Check sheet for the modelled part. Datum: model origin and axes. Units: mm. A direction names the side the tool comes from. Give positions to 0.01 mm unless a question says otherwise; leave off trailing zeros. Write each loop counter-clockwise with the first axis right and the second up, starting at its lowest first coordinate (ties: lowest second). Pieces come first, ordered by that corner, then holes. Notation, with made-up numbers: (7.5, 52.25) -> (59.5, 52.25) arc R30 cw to (59.5, 77.25) -> close; hole circle Ø5 at (8.5, 31). An arc over 180 degrees is marked (long way). Use a Markdown table: item, result. Add a question column.
1. Cross-section at D-D (y = 160.5). Enter the section's corners in (x, z), then the cut area to 3 significant figures.
2. Cross-section at A-A (z = 0). Enter the section's corners in (x, y).
3. Gauge pin test, flat ends, axial feed: P1, Ø1.5, axis at x = 70, y = 53, coming from the +Z side; P2, Ø3, axis at x = -80, y = 63.5, coming from the -Z side; P3, Ø5.5, axis at x = -80, z = 46.5, coming from the +Y side; P4, Ø1.5, axis at x = 81.5, z = 18, coming from the -Y side. Record the tip position at first contact, or that the pin passes through.
4. Cross-section at B-B (x = 0). Enter the section's corners in (y, z).
5. Cross-section at C-C (y = 209). Enter the section's corners in (x, z), then the cut area to 3 significant figures.
6. Release check for a two-part mould opening along X. For faces 1 (the cylindrical face through (-15.456, 224.956, -20.157)), 2 (the cylindrical face through (0.372, 29.58, -118.492)), 3 (the flat face through (-72.335, 63.131, 41.852)), 4 (the cylindrical face through (77.38, 29.58, -43.77)) record: released by +X, released by -X, zero draft, split by the parting line, or undercut.
7. Set-up check for faces 5 (the flat face through (-67, 30, 71.947)), 6 (the flat face through (66, 30, 71.947)), 7 (the flat face through (-81, 66.35, 46)), 8 (the cylindrical face through (22.89, 153.67, -72.68)): record each of +Z, -Z, +X, -X, +Y, -Y from which the full face is reachable in a straight line by a thin tool's end or side.
8. Scan lines: probe 1 along X at (y, z) = (219.5, 0); probe 2 along Y at (x, z) = (-63, 53.5); probe 3 along Y at (x, z) = (-7, -4). Record each from-to range of solid material in increasing order. Write a range as [from, to].
from build123d import *

# Parameters (mm, degrees)
BOSS_EXTRUDE1_DEPTH = 60
BOSS_EXTRUDE2_DEPTH = 6.35
SKETCH3_R           = 76.2
BOSS_EXTRUDE3_DEPTH = 250
SKETCH4_R           = 25.4
CUT_EXTRUDE1_DEPTH  = 50.8


with BuildPart() as part:
    # Sketch1 → Boss-Extrude1 (new body)
    with BuildSketch(Plane(origin=(0, 0, 0), x_dir=(1, 0, 0), z_dir=(0, 1, 0))):
        with BuildLine():
            ThreePointArc((-36.198972693, 81.196332281), (-76.989658396, 44.45), (-88.417572796, -9.248936198))
            Line((-88.417572796, -9.248936198), (-102.619500233, -33.847396084))
            ThreePointArc((-102.619500233, -33.847396084), (-102.619500233, -59.247396084), (-80.622454977, -71.947396084))
            Line((-80.622454977, -71.947396084), (-52.218600103, -71.947396084))
            ThreePointArc((-52.218600103, -71.947396084), (0, -88.9), (52.218600103, -71.947396084))
            Line((52.218600103, -71.947396084), (80.622454977, -71.947396084))
            ThreePointArc((80.622454977, -71.947396084), (102.619500233, -59.247396084), (102.619500233, -33.847396084))
            Line((102.619500233, -33.847396084), (88.417572796, -9.248936198))
            ThreePointArc((88.417572796, -9.248936198), (76.989658396, 44.45), (36.198972693, 81.196332281))
            Line((36.198972693, 81.196332281), (21.997045256, 105.794792168))
            ThreePointArc((21.997045256, 105.794792168), (0, 118.494792168), (-21.997045256, 105.794792168))
            Line((-21.997045256, 105.794792168), (-36.198972693, 81.196332281))
        make_face()
        with BuildLine():
            ThreePointArc((-75.786490968, -7.927659598), (-65.991135768, 38.1), (-31.02769088, 69.596856241))
            ThreePointArc((-31.02769088, 69.596856241), (0, 76.2), (31.02769088, 69.596856241))
            ThreePointArc((31.02769088, 69.596856241), (63.916938463, 41.485720163), (76.2, 0))
            ThreePointArc((76.2, 0), (76.096552523, -3.969218324), (75.786490968, -7.927659598))
            ThreePointArc((75.786490968, -7.927659598), (65.991135768, -38.1), (44.758800089, -61.669196643))
            ThreePointArc((44.758800089, -61.669196643), (0, -76.2), (-44.758800089, -61.669196643))
            ThreePointArc((-44.758800089, -61.669196643), (-65.991135768, -38.1), (-75.786490968, -7.927659598))
        make_face(mode=Mode.SUBTRACT)
    extrude(amount=BOSS_EXTRUDE1_DEPTH)

    # Sketch2 → Boss-Extrude2 (add)
    with BuildSketch(Plane(origin=(0, 60, 0), x_dir=(1, 0, 0), z_dir=(0, 1, 0))):
        Polygon((-69.623932349, -46.547396084), (-75.123193663, -37.022396084), (-86.121716291, -37.022396084), (-91.620977605, -46.547396084), (-86.121716291, -56.072396084), (-75.123193663, -56.072396084), align=None)
    extrude(amount=BOSS_EXTRUDE2_DEPTH)

    # Sketch3 → Boss-Extrude3 (add)
    with BuildSketch(Plane.XZ):
        with Locations(Location((0, 0, 0), (0, 0, 270))):
            Circle(SKETCH3_R)
    extrude(amount=-BOSS_EXTRUDE3_DEPTH)

    # Sketch4 → Cut-Extrude1 (cut)
    with BuildSketch(Plane(origin=(0, 250, 0), x_dir=(1, 0, 0), z_dir=(0, 1, 0))):
        with Locations(Location((0, 0, 0), (0, 0, 270))):
            Circle(SKETCH4_R)
    extrude(amount=-CUT_EXTRUDE1_DEPTH, mode=Mode.SUBTRACT)


solid = part.part
Worked answers:
| question | item | result |
|---|---|---|
| 1 | outline | circle Ø152.4 at (0, 0) |
| 1 | area | 18,200 mm² |
| 2 | outline | (-88.9, 0) -> (88.9, 0) -> (88.9, 60) -> (76.2, 60) -> (76.2, 250) -> (25.4, 250) -> (25.4, 199.2) -> (-25.4, 199.2) -> (-25.4, 250) -> (-76.2, 250) -> (-76.2, 60) -> (-88.9, 60) -> close |
| 3 | P1 | stops at z = 71.95 |
| 3 | P2 | stops at z = 37.02 |
| 3 | P3 | stops at y = 66.35 |
| 3 | P4 | stops at y = 0 |
| 4 | outline | (0, -118.49) -> (60, -118.49) -> (60, -76.2) -> (250, -76.2) -> (250, -25.4) -> (199.2, -25.4) -> (199.2, 25.4) -> (250, 25.4) -> (250, 76.2) -> (60, 76.2) -> (60, 88.9) -> (0, 88.9) -> close |
| 5 | outline | circle Ø152.4 at (0, 0); hole circle Ø50.8 at (0, 0) |
| 5 | area | 16,200 mm² |
| 6 | face 1 | undercut |
| 6 | face 2 | split by the parting line |
| 6 | face 3 | undercut |
| 6 | face 4 | released by +X |
| 7 | face 5 | +Z, -X, +Y, -Y |
| 7 | face 6 | +Z, +X, +Y, -Y |
| 7 | face 7 | +Z, -X, +Y |
| 7 | face 8 | +Y |
| 8 | probe 1 | x = [-76.2, -25.4], [25.4, 76.2] |
| 8 | probe 2 | y = [0, 60] |
| 8 | probe 3 | y = [0, 199.2] |
